Could you check a few things on this model? Use its own coordinates, in mm. Face numbers are marked on the shaded views. A direction names the side the tool comes from. Give positions to 0.01 mm unless a question says otherwise; leave off trailing zeros. Order: outer loops, then holes, each group sorted by start corner. A loop starts at its lowest first (then second) coordinate and runs counter-clockwise, first axis right, second up. Notation, with made-up numbers: M 61.25,58.25 L 110.25,58.25 A30 cw 110.25,86.25 Z; hole C 64.5,-10.75 d4. An arc over 180 degrees is marked long. Use a Markdown table: item, result. Add a question column.
Item 1: I'm going to push flat-ended pins straight in: pin 1 Ø12 at (x, y) = (0, 28) entering from -Z; pin 2 Ø5 at (x, y) = (10.5, 25) entering from +Z; pin 3 Ø8 at (x, z) = (1, -10.5) entering from +Y; pin 4 Ø4 at (x, z) = (4.5, 14.5) entering from -Y. Where does each tip first touch, or does it pass through?
Item 2: Suppose I cut it at C-C on y = 13.5. Write out the boundary of the cut face in (x, z), plus the area to 3 significant figures.
Item 3: Suppose I cut it at B-B on x = -5. Write out the boundary of the cut face in (y, z), plus the area to 3 significant figures.
Item 4: If I drill on L1, parallel to X at y = 25, z = -5.5; L2, parallel to Y at x = -1, z = 2.5; L3, parallel to Z at x = -8.5, y = 19, over which ranges is the centre line in solid material (lowest first)? Write a range as from..to.
Item 5: Suppose I cut it at D-D on x = -11.5. Write out the boundary of the cut face in (y, z), plus the area to 3 significant figures.
Item 6: Suppose I cut it at A-A on z = -12. Write out the boundary of the cut face in (x, y).
Item 7: For the marked faces 1 and 2, which set-ups out of +Z, -Z, +X, -X, +Y, -Y let a thin tool reach every point of the face, with its end or its side?
from build123d import *

# Parameters (mm, degrees)
SKETCH1_W           = 38.1
SKETCH1_H           = 38.1
BOSS_EXTRUDE1_DEPTH = 2.54
SKETCH2_W           = 19.05
SKETCH2_H           = 19.05
BOSS_EXTRUDE2_DEPTH = 31.75
BOSS_EXTRUDE3_DEPTH = 3.81
BOSS_EXTRUDE4_DEPTH = 3.81
SKETCH5_W           = 15.24
SKETCH5_H           = 15.24
CUT_EXTRUDE1_DEPTH  = 31.75
CHAMFER5_SIZE       = 6.35


with BuildPart() as part:
    # Sketch1 → Boss-Extrude1 (new body)
    with BuildSketch(Plane(origin=(0, 0, 0), x_dir=(1, 0, 0), z_dir=(0, 1, 0))):
        Rectangle(SKETCH1_W, SKETCH1_H)
    extrude(amount=BOSS_EXTRUDE1_DEPTH)

    # Sketch2 → Boss-Extrude2 (add)
    with BuildSketch(Plane(origin=(0, 2.54, 0), x_dir=(1, 0, 0), z_dir=(0, 1, 0))):
        with Locations((-9.525, -9.525)):
            Rectangle(SKETCH2_W, SKETCH2_H)
    extrude(amount=BOSS_EXTRUDE2_DEPTH)

    # Sketch3 → Boss-Extrude3 (add)
    with BuildSketch(Plane.XY.offset(19.05)):
        Polygon((0, 34.29), (19.05, 2.54), (0, 2.54), align=None)
    extrude(amount=-BOSS_EXTRUDE3_DEPTH)

    # Sketch4 → Boss-Extrude4 (add)
    with BuildSketch(Plane.ZY.offset(19.05)):
        Polygon((0, 34.29), (0, 2.54), (-19.05, 2.54), align=None)
    extrude(amount=-BOSS_EXTRUDE4_DEPTH)

    # Sketch5 → Cut-Extrude1 (cut)
    with BuildSketch(Plane(origin=(0, 34.29, 0), x_dir=(1, 0, 0), z_dir=(0, 1, 0))):
        with Locations((-7.62, -7.62)):
            Rectangle(SKETCH5_W, SKETCH5_H)
    extrude(amount=-CUT_EXTRUDE1_DEPTH, mode=Mode.SUBTRACT)

    # Chamfer5
    chamfer5_edges = [part.edges().sort_by_distance(p)[0] for p in [
        (1.905, 2.54, 15.24),
        (-15.24, 2.54, -1.905),
    ]]
    chamfer(chamfer5_edges, length=CHAMFER5_SIZE)


solid = part.part
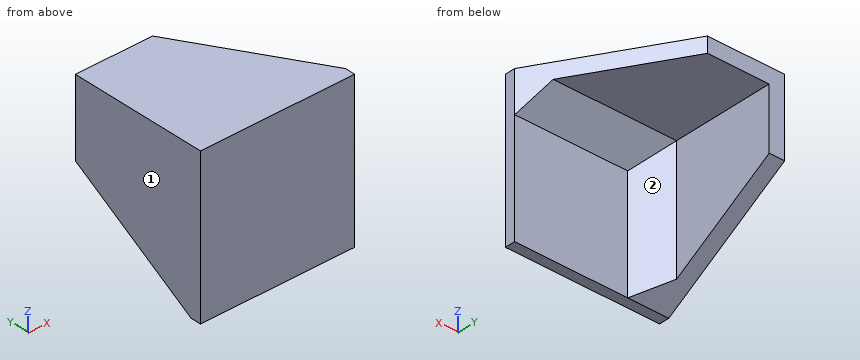
Findings below:
| question | item | result |
|---|---|---|
| 1 | pin 1 | stops at z = 15.24 |
| 1 | pin 2 | passes through |
| 1 | pin 3 | stops at y = 2.54 |
| 1 | pin 4 | stops at y = 0 |
| 2 | outline | M -19.05,-12.47 L -15.24,-12.47 L -15.24,15.24 L 12.47,15.24 L 12.47,19.05 L -19.05,19.05 Z |
| 2 | area | 226 mm^2 |
| 3 | outline | M 0,-19.05 L 2.54,-19.05 L 2.54,8.89 L 8.89,15.24 L 34.29,15.24 L 34.29,19.05 L 0,19.05 Z |
| 3 | area | 238 mm^2 |
| 4 | L1 | x = -19.05..-15.24 |
| 4 | L2 | y = 0..2.54 |
| 4 | L3 | z = 15.24..19.05 |
| 5 | outline | M 0,-19.05 L 2.54,-19.05 L 5.15,-17.48 L 5.15,11.5 L 8.89,15.24 L 34.29,15.24 L 34.29,19.05 L 0,19.05 Z |
| 5 | area | 312 mm^2 |
| 6 | outline | M -19.05,0 L 19.05,0 L 19.05,2.54 L -8.89,2.54 L -15.24,8.89 L -15.24,14.29 L -19.05,14.29 Z |
| 7 | face 1 | +Z, -Z, -X, +Y, -Y |
| 7 | face 2 | -Z, +X, +Y |
